```python
from build123d import *

# Parameters (mm, degrees)
F1_DEPTH    = 23
F2_R        = 4
F3_DEPTH    = 35.0010001
F5_DEPTH    = 32
F6_SIZE     = 1
F7_T1_DEPTH = 28.1474867513
F8_T1_DEPTH = 33.2835617863
F9_SIZE     = 3


# Not quite as in the source:
# - a fillet or chamfer that OpenCascade refuses, or shapes differently, is made with other operations: its cross-section is extruded or revolved along the edge and cut away or added


with BuildPart() as f1:
    # F0 (on Front) → F1 (new body)
    with BuildSketch(Plane.XZ):
        with BuildLine():
            Line((-35, 0), (0, 0))
            Line((0, 0), (0, 21))
            add(Edge.make_bspline(
                [(-35, 19), (-12.9749150947, 19.5710677654), (-12.9749150947, 20.0476832688), (0, 21)],
                knots=[0, 0, 0, 0, 35.0570962859, 35.0570962859, 35.0570962859, 35.0570962859], degree=3))
            Line((-35, 19), (-35, 0))
        make_face()
    extrude(amount=F1_DEPTH)

    # F2 (on Right) → F3 (cut, through all)
    with BuildSketch(Plane.YZ):
        with Locations((-9, 9.5)):
            Circle(F2_R)
    extrude(amount=-F3_DEPTH, mode=Mode.SUBTRACT)

    # F4 (on Right) → F5 (cut)
    with BuildSketch(Plane.YZ):
        Polygon((-5.225094273, 3.0128264948), (-1.4944900823, 9.5255775039), (-5.2693958093, 16.012751009), (-12.774905727, 15.9871735052), (-16.5055099177, 9.4744224961), (-12.7306041907, 2.987248991), align=None)
    extrude(amount=-F5_DEPTH, mode=Mode.SUBTRACT)

    # F6
    f6_edges = [f1.edges().sort_by_distance(p)[0] for p in [
        (0, -11.5, 0),
    ]]
    chamfer(f6_edges, length=F6_SIZE)

    # F7: chamfer of 1 on 1 edges, made by hand

    # F7_s2 → F7_t1 (cut)
    with BuildSketch(Plane.XZ.offset(-2.5737433757)):
        with BuildLine():
            Line((0.0293272632, 19.9718445491), (-1.0284200625, 20.9529152979))
            Line((-1.0284200625, 20.9529152979), (-1.0299222717, 20.9728588023))
            ThreePointArc((-1.0299222717, 20.9728588023), (-0.5146246013, 20.9820315927), (-0.0014639972, 21.0199463458))
            Line((-0.0014639972, 21.0199463458), (0.02, 21))
            ThreePointArc((0.02, 21), (0.02, 20.4859222745), (0.0493272632, 19.9718445491))
            Line((0.0493272632, 19.9718445491), (0.0293272632, 19.9718445491))
        make_face()
    extrude(amount=F7_T1_DEPTH, mode=Mode.SUBTRACT)

    # F8: chamfer of 2 on 1 edges, made by hand

    # F8_s2 → F8_t1 (cut)
    with BuildSketch(Plane.XZ.offset(-5.1417808931)):
        with BuildLine():
            Line((-35.0557899395, 16.944044455), (-32.9477944744, 19.1104787201))
            Line((-32.9477944744, 19.1104787201), (-32.9488880075, 19.1504637697))
            ThreePointArc((-32.9488880075, 19.1504637697), (-33.974209491, 19.0669652644), (-35.001036774, 19.0399865615))
            Line((-35.001036774, 19.0399865615), (-35.04, 19))
            ThreePointArc((-35.04, 19), (-35.04, 17.9720222275), (-35.0957899395, 16.944044455))
            Line((-35.0957899395, 16.944044455), (-35.0557899395, 16.944044455))
        make_face()
    extrude(amount=F8_T1_DEPTH, mode=Mode.SUBTRACT)

    # F9
    f9_edges = [f1.edges().sort_by_distance(p)[0] for p in [
        (-35, -11.5, 0),
    ]]
    chamfer(f9_edges, length=F9_SIZE)


solid = f1.part
```
The model under review builds one solid part; all positions refer to its coordinate system, in mm. A direction names the side the tool comes from. Give positions to 0.01 mm unless a question says otherwise; leave off trailing zeros. Write each loop counter-clockwise with the first axis right and the second up, starting at its lowest first coordinate (ties: lowest second). Pieces come first, ordered by that corner, then holes. Notation, with made-up numbers: (70.25, 84.5) -> (110.25, 84.5) arc R25 ccw to (110.25, 106.5) -> close; hole circle Ø10 at (40.25, 32.5). An arc over 180 degrees is marked (long way). Put each result on its own line as item: value.
(1) We need section A-A, the plane z = 6.25. Give the boundary of the cut face in (x, y), and give its area (3 significant figures).
Results are:
outline: (-35, -23) -> (0, -23) -> (0, -14.63) -> (-32, -14.63) -> (-32, -11.33) -> (-35, -11.33) -> close; (-35, -6.67) -> (-32, -6.67) -> (-32, -3.37) -> (0, -3.37) -> (0, 0) -> (-35, 0) -> close
area: 431 mm²
(2) We need section B-B, the plane z = 3.75. Give the boundary of the cut face in (x, y).
Results are:
outline: (-35, -23) -> (0, -23) -> (0, -13.17) -> (-32, -13.17) -> (-32, -4.8) -> (0, -4.8) -> (0, 0) -> (-35, 0) -> close
(3) To check wall thickness, follow probe 1 along X at (y, z) = (-5, 5.25); probe 2 along Z at (x, y) = (-17, -14.75); probe 3 along Y at (x, z) = (-29, 3.25). State the ranges of each line that lie inside material, in increasing order. Write a range as from..to.
Results are:
probe 1: -35..-32
probe 2: 0..6.46, 12.54..19.67
probe 3: -23..-12.88, -5.09..0
(4) We need section C-C, the plane z = 12. Give the boundary of the cut face in (x, y).
Results are:
outline: (-35, -23) -> (0, -23) -> (0, -15.06) -> (-32, -15.06) -> (-32, -12.12) -> (-35, -12.12) -> close; (-35, -5.88) -> (-32, -5.88) -> (-32, -2.93) -> (0, -2.93) -> (0, 0) -> (-35, 0) -> close
(5) Tool access review of faces 1 (the flat face through (-34, -11, 2)), 2 (the flat face through (-15.8, -3.4, 6.2)): name each direction out of +Z, -Z, +X, -X, +Y, -Y from which nothing blocks a thin tool from reaching the whole face with its end or side.
Results are:
face 1: -Z, -X, +Y, -Y
face 2: +X
(6) The part is to be moulded in two halves that separate along Z. For faces 3 (the flat face through (-18, -23, 11)), 4 (the flat face through (-34.02, -11.34, 18.01)), 5 (the flat face through (-32, -5.8, 12.5)), 6 (the flat face through (-0.5, -11.3, 0.5)), say which applies: pulls with the +Z half, pulls with the -Z half, needs draft (parallel to the pull), parting line crosses it, or undercut.
Results are:
face 3: needs draft
face 4: pulls with the +Z half
face 5: undercut
face 6: pulls with the -Z half
(7) For pin 1 Ø6.5 at (y, z) = (-11.5, 9) entering from +X; pin 2 Ø8 at (x, y) = (-29.5, -15.5) entering from +Z, all flat-tipped, find the tip position at first contact; note any pin that passes through.
Results are:
pin 1: x = -32
pin 2: z = 19.29
